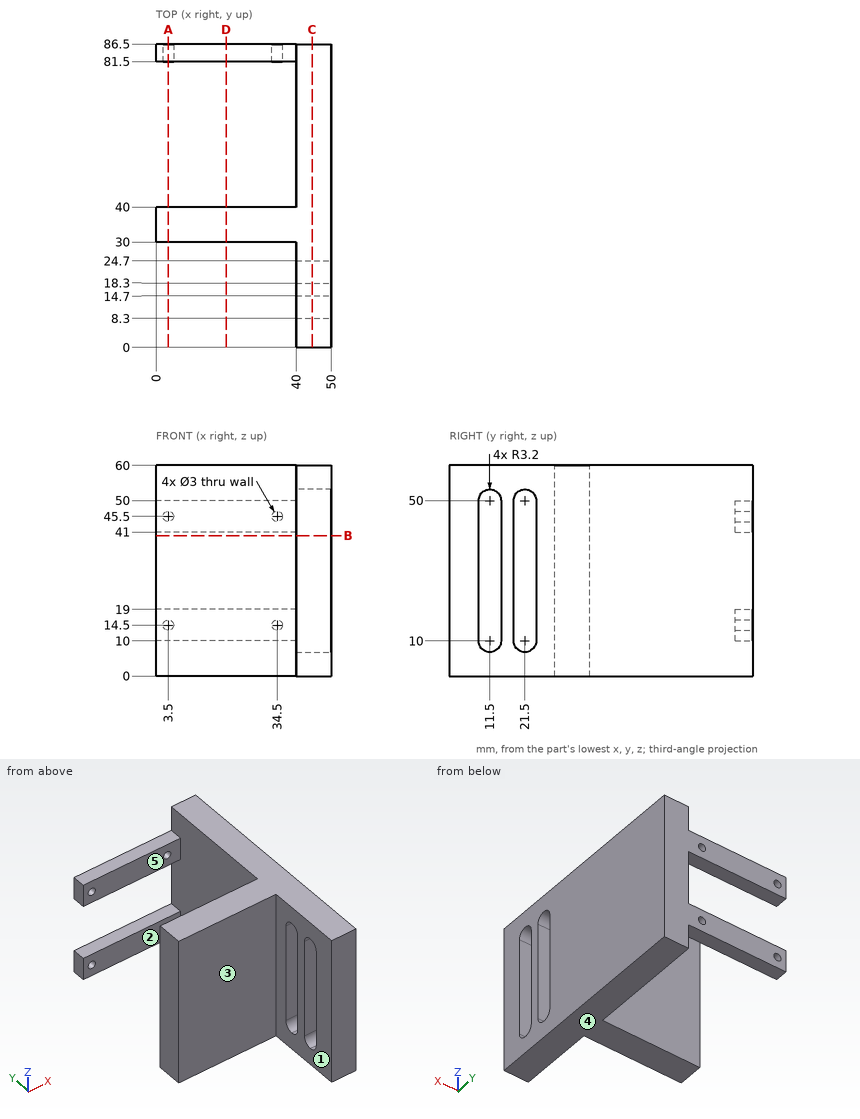
Geometry: see drawing. Coordinates: mm, zero at the bounding-box minimum. A direction names the side the tool comes from. Round coordinates to 2 decimals unless told otherwise and drop trailing zeros. Loops run counter-clockwise (first coordinate to the right, second up) from the corner with the lowest first, then second, coordinate; pieces in that order, holes last. Notation, with made-up numbers: (-17, 14) -> (24, 14) arc R28 cw to (24, 48) -> close; hole circle Ø3 at (77, -16). An arc over 180 degrees is marked (long way). One line per question, with ' | ' between items. Start each with the question number.
1. Section D-D on x = 20. Output: boundary loops of the cut face in (y, z), and give its area (3 significant figures).
2. Mould query, pull axis Y, two halves, no side actions, for the marked faces 1, 2 and 3. Classes: pulls with the +Y half, pulls with the -Y half, needs draft (parallel to the pull), parting line crosses it, or undercut.
3. Set-up query: the marked faces 4 and 5. Return all of +Z, -Z, +X, -X, +Y, -Y with unobstructed straight access to the full face (end or side cutting, diameter ignored); none if empty.
4. Contact query for flat-ended pins moving along their axis: pin 1 (2.5 mm diameter, centred on x = 34.5, z = 14.5, fed in from +Y); pin 2 (10 mm diameter, centred on y = 20, z = 25.5, fed in from -X); pin 3 (2.5 mm diameter, centred on x = 26.5, z = 46.5, fed in from -Y). Output: stop coordinate, or through.
5. Line query: line 1 along Y through (x, z) = (45.5, 18); line 2 along Z through (x, y) = (3.5, 85.2); line 3 along X through (y, z) = (85.1, 14.5). Output: solid intervals per line, ascending. Write a range as [from, to].
6. Section B-B on z = 40. Output: boundary loops of the cut face in (x, y).
7. Section A-A on x = 3.5. Output: boundary loops of the cut face in (y, z).
8. Section C-C on x = 44.5. Output: boundary loops of the cut face in (y, z), and give its area (3 significant figures).
Returned:
1) outline: (30, 0) -> (40, 0) -> (40, 60) -> (30, 60) -> close; (81.5, 10) -> (86.5, 10) -> (86.5, 19) -> (81.5, 19) -> close; (81.5, 41) -> (86.5, 41) -> (86.5, 50) -> (81.5, 50) -> close | area: 690 mm2
2) face 1: needs draft | face 2: undercut | face 3: pulls with the -Y half
3) face 4: -Z, +X, -X, +Y, -Y | face 5: +Z, -Z, -X
4) pin 1: stops at y = 40 | pin 2: stops at x = 40 | pin 3: stops at y = 30
5) line 1: y = [0, 8.3], [14.7, 18.3], [24.7, 86.5] | line 2: z = [10, 13], [16, 19], [41, 44], [47, 50] | line 3: x = [0, 2], [5, 33], [36, 50]
6) outline: (0, 30) -> (40, 30) -> (40, 24.7) -> (50, 24.7) -> (50, 86.5) -> (40, 86.5) -> (40, 40) -> (0, 40) -> close; (40, 0) -> (50, 0) -> (50, 8.3) -> (40, 8.3) -> close; (40, 14.7) -> (50, 14.7) -> (50, 18.3) -> (40, 18.3) -> close
7) outline: (30, 0) -> (40, 0) -> (40, 60) -> (30, 60) -> close; (81.5, 10) -> (86.5, 10) -> (86.5, 13) -> (81.5, 13) -> close; (81.5, 16) -> (86.5, 16) -> (86.5, 19) -> (81.5, 19) -> close; (81.5, 41) -> (86.5, 41) -> (86.5, 44) -> (81.5, 44) -> close; (81.5, 47) -> (86.5, 47) -> (86.5, 50) -> (81.5, 50) -> close
8) outline: (0, 0) -> (86.5, 0) -> (86.5, 60) -> (0, 60) -> close; hole (8.3, 10) arc R3.2 ccw to (14.7, 10) -> (14.7, 50) arc R3.2 ccw to (8.3, 50) -> close; hole (18.3, 10) arc R3.2 ccw to (24.7, 10) -> (24.7, 50) arc R3.2 ccw to (18.3, 50) -> close | area: 4,610 mm2
